Design review of the part built by this model. Coordinates are the model's own, in mm. A direction names the side the tool comes from. Give positions to 0.01 mm unless a question says otherwise; leave off trailing zeros. Write each question's results on one line, items separated by ' | '. Start each with the question number.
from build123d import *

# Parameters (mm, degrees)
BOSS_EXTRUDE1_DEPTH = 3.175
BOSS_EXTRUDE2_DEPTH = 3.175
BOSS_EXTRUDE3_DEPTH = 3.175


with BuildPart() as part:
    # Sketch1 → Boss-Extrude1 (new body)
    with BuildSketch(Plane.XY):
        with BuildLine():
            Line((0, 0), (0, 35.921024484))
            ThreePointArc((0, 35.921024484), (-25.4, 25.4), (-35.921024484, 0))
            Line((-35.921024484, 0), (0, 0))
        make_face()
    extrude(amount=BOSS_EXTRUDE1_DEPTH)

    # Sketch2 → Boss-Extrude2 (add)
    with BuildSketch(Plane(origin=(0, 0, 0), x_dir=(0, 0, -1), z_dir=(1, 0, 0))):
        with BuildLine():
            Line((0, 0), (25.4, 0))
            Line((25.4, 0), (25.4, 17.145))
            ThreePointArc((25.4, 17.145), (15.793187578, 30.717442473), (0, 35.921024484))
            Line((0, 35.921024484), (-3.175, 35.921024484))
            Line((-3.175, 35.921024484), (-3.175, 0))
            Line((-3.175, 0), (0, 0))
        make_face()
    extrude(amount=BOSS_EXTRUDE2_DEPTH)

    # Sketch3 → Boss-Extrude3 (add)
    with BuildSketch(Plane.XZ):
        with BuildLine():
            Line((0, -25.4), (-17.145, -25.4))
            ThreePointArc((-17.145, -25.4), (-30.717442473, -15.793187578), (-35.921024484, 0))
            Line((-35.921024484, 0), (-35.921024484, 3.175))
            Line((-35.921024484, 3.175), (3.175, 3.175))
            Line((3.175, 3.175), (3.175, -25.4))
            Line((3.175, -25.4), (0, -25.4))
        make_face()
    extrude(amount=BOSS_EXTRUDE3_DEPTH)

    # Chamfer1
    # the kernel refuses this chamfer: 2.032 mm, written as the material it takes off along each edge
    with BuildSketch(Plane(origin=(1.820333333, 34.566357818, 1.820333333), x_dir=(0, -0.7071067811865468, 0.7071067811865481), z_dir=(0.5773502691896253, 0.5773502691896264, 0.5773502691896256))) as chamfer1_piece_1:
        Polygon((-1.436840979, -0.829560526), (1.436840979, -0.829560526), (0, 1.659121052), align=None)
    extrude(amount=2.580986643, mode=Mode.SUBTRACT)
    with BuildSketch(Plane(origin=(1.820333333, -1.820333333, -24.045333333), x_dir=(-0.7071067811865476, 0, -0.7071067811865476), z_dir=(0.5773502691896256, -0.577350269189626, -0.5773502691896256)), Plane(origin=(1.820333333, -1.820333333, 1.820333333), x_dir=(0.7071067811865476, 0, -0.7071067811865474), z_dir=(0.5773502691896254, -0.577350269189626, 0.577350269189626)), Plane(origin=(-34.566357818, -1.820333333, 1.820333333), x_dir=(0.7071067811865468, 0, 0.7071067811865481), z_dir=(-0.5773502691896263, -0.5773502691896255, 0.5773502691896255))) as chamfer1_piece_2:
        Polygon((-1.436840979, 0.829560526), (1.436840979, 0.829560526), (0, -1.659121052), align=None)
    extrude(amount=2.580986643, mode=Mode.SUBTRACT)
    with BuildSketch(Plane(origin=(0, 0, 3.175), x_dir=(0, 1, 0), z_dir=(1, 0, 0))) as chamfer1_piece_3:
        with BuildLine():
            Line((35.978498123, -2.089473639), (33.831550845, 0.057473639))
            Line((33.831550845, 0.057473639), (33.831550845, 0.098113639))
            ThreePointArc((33.831550845, 0.098113639), (34.876287665, 0.04064), (35.921024484, 0.04064))
            Line((35.921024484, 0.04064), (35.961664484, 0))
            ThreePointArc((35.961664484, 0), (35.961664484, -1.04473682), (36.019138123, -2.089473639))
            Line((36.019138123, -2.089473639), (35.978498123, -2.089473639))
        make_face()
    revolve(axis=Axis((0, 0, 3.175), (0, 0, 1)), revolution_arc=90, mode=Mode.SUBTRACT)
    with BuildSketch(Plane(origin=(0, 35.921024484, 3.175), x_dir=(0, -0.9996219169112968, 0.027495876610586455), z_dir=(1, 0, 0)), Plane(origin=(-35.921024484, -3.175, 0), x_dir=(0.9996219169112968, -0.027495876610586455, 0), z_dir=(0, 0, 1))) as chamfer1_piece_4:
        with BuildLine():
            Line((2.090263933, 0), (-0.114903819, 2.087103356))
            Line((-0.114903819, 2.087103356), (-0.155528453, 2.085985924))
            ThreePointArc((-0.155528453, 2.085985924), (-0.069350589, 1.04322439), (-0.040624635, -0.001117432))
            Line((-0.040624635, -0.001117432), (0.001117432, -0.040624635))
            ThreePointArc((0.001117432, -0.040624635), (1.045459255, -0.01189868), (2.091381365, -0.040624635))
            Line((2.091381365, -0.040624635), (2.090263933, 0))
        make_face()
    extrude(amount=8.400659832, mode=Mode.SUBTRACT)
    with BuildSketch(Plane(origin=(3.175, 22.370659832, -25.4), x_dir=(0.027495876610586455, 0, 0.9996219169112968), z_dir=(0, -1, 0))) as chamfer1_piece_5:
        with BuildLine():
            Line((2.090263933, 0), (-0.114903819, 2.087103356))
            Line((-0.114903819, 2.087103356), (-0.155528453, 2.085985924))
            ThreePointArc((-0.155528453, 2.085985924), (-0.069350589, 1.04322439), (-0.040624635, -0.001117432))
            Line((-0.040624635, -0.001117432), (0.001117432, -0.040624635))
            ThreePointArc((0.001117432, -0.040624635), (1.045459255, -0.01189868), (2.091381365, -0.040624635))
            Line((2.091381365, -0.040624635), (2.090263933, 0))
        make_face()
    extrude(amount=30.771319663, mode=Mode.SUBTRACT)
    with BuildSketch(Plane(origin=(3.175, 9.352591527, 0), x_dir=(0, 0.1007624019843993, -0.9949105177584235), z_dir=(0, -0.9949105177584235, -0.1007624019843993))) as chamfer1_piece_6:
        with BuildLine():
            Line((24.478959318, 0.057473639), (26.625906597, -2.089473639))
            Line((26.625906597, -2.089473639), (26.666546597, -2.089473639))
            ThreePointArc((26.666546597, -2.089473639), (26.609072957, -1.04473682), (26.609072957, 0))
            Line((26.609072957, 0), (26.568432957, 0.04064))
            ThreePointArc((26.568432957, 0.04064), (25.523696138, 0.04064), (24.478959318, 0.098113639))
            Line((24.478959318, 0.098113639), (24.478959318, 0.057473639))
        make_face()
    revolve(axis=Axis((3.175, 9.352591527, 0), (1, 0, 0)), revolution_arc=84.216925348, mode=Mode.SUBTRACT)
    with BuildSketch(Plane(origin=(3.175, 35.921024484, 0), x_dir=(0.027495876610586455, -0.9996219169112968, 0), z_dir=(0, 0, 1)), Plane(origin=(-35.921024484, 0, 3.175), x_dir=(0.9996219169112968, 0, 0.027495876610586455), z_dir=(0, -1, 0))) as chamfer1_piece_7:
        with BuildLine():
            Line((2.090263933, 0), (-0.114903819, -2.087103356))
            Line((-0.114903819, -2.087103356), (-0.155528453, -2.085985924))
            ThreePointArc((-0.155528453, -2.085985924), (-0.069350589, -1.04322439), (-0.040624635, 0.001117432))
            Line((-0.040624635, 0.001117432), (0.001117432, 0.040624635))
            ThreePointArc((0.001117432, 0.040624635), (1.045459255, 0.01189868), (2.091381365, 0.040624635))
            Line((2.091381365, 0.040624635), (2.090263933, 0))
        make_face()
    extrude(amount=8.400659832, mode=Mode.SUBTRACT)
    with BuildSketch(Plane(origin=(3.175, -8.400659832, 3.175), x_dir=(-0.9996219169112968, 0, 0.027495876610586435), z_dir=(0, 1, 0)), Plane(origin=(-41.146684316, -3.175, 3.175), x_dir=(0, 0.9996219169112968, 0.027495876610586435), z_dir=(1, 0, 0))) as chamfer1_piece_8:
        with BuildLine():
            Line((2.090263933, 0), (-0.114903819, -2.087103356))
            Line((-0.114903819, -2.087103356), (-0.155528453, -2.085985924))
            ThreePointArc((-0.155528453, -2.085985924), (-0.069350589, -1.04322439), (-0.040624635, 0.001117432))
            Line((-0.040624635, 0.001117432), (0.001117432, 0.040624635))
            ThreePointArc((0.001117432, 0.040624635), (1.045459255, 0.01189868), (2.091381365, 0.040624635))
            Line((2.091381365, 0.040624635), (2.090263933, 0))
        make_face()
    extrude(amount=49.547344147, mode=Mode.SUBTRACT)
    with BuildSketch(Plane(origin=(8.400659832, -3.175, -25.4), x_dir=(0, 0.9996219169112968, -0.027495876610585585), z_dir=(-1, 0, 0))) as chamfer1_piece_9:
        with BuildLine():
            Line((2.090263933, 0), (-0.114903819, -2.087103356))
            Line((-0.114903819, -2.087103356), (-0.155528453, -2.085985924))
            ThreePointArc((-0.155528453, -2.085985924), (-0.069350589, -1.04322439), (-0.040624635, 0.001117432))
            Line((-0.040624635, 0.001117432), (0.001117432, 0.040624635))
            ThreePointArc((0.001117432, 0.040624635), (1.045459255, 0.01189868), (2.091381365, 0.040624635))
            Line((2.091381365, 0.040624635), (2.090263933, 0))
        make_face()
    extrude(amount=30.771319663, mode=Mode.SUBTRACT)
    with BuildSketch(Plane(origin=(3.175, -3.175, 8.400659832), x_dir=(0.027495876610586435, 0.9996219169112968, 0), z_dir=(0, 0, -1))) as chamfer1_piece_10:
        with BuildLine():
            Line((2.090263933, 0), (-0.114903819, -2.087103356))
            Line((-0.114903819, -2.087103356), (-0.155528453, -2.085985924))
            ThreePointArc((-0.155528453, -2.085985924), (-0.069350589, -1.04322439), (-0.040624635, 0.001117432))
            Line((-0.040624635, 0.001117432), (0.001117432, 0.040624635))
            ThreePointArc((0.001117432, 0.040624635), (1.045459255, 0.01189868), (2.091381365, 0.040624635))
            Line((2.091381365, 0.040624635), (2.090263933, 0))
        make_face()
    extrude(amount=39.026319663, mode=Mode.SUBTRACT)
    with BuildSketch(Plane(origin=(-9.352591527, -3.175, 0), x_dir=(-0.1007624019843981, 0, -0.9949105177584237), z_dir=(0.9949105177584237, 0, -0.1007624019843981))) as chamfer1_piece_11:
        with BuildLine():
            Line((26.625906597, 2.089473639), (24.478959318, -0.057473639))
            Line((24.478959318, -0.057473639), (24.478959318, -0.098113639))
            ThreePointArc((24.478959318, -0.098113639), (25.523696138, -0.04064), (26.568432957, -0.04064))
            Line((26.568432957, -0.04064), (26.609072957, 0))
            ThreePointArc((26.609072957, 0), (26.609072957, 1.04473682), (26.666546597, 2.089473639))
            Line((26.666546597, 2.089473639), (26.625906597, 2.089473639))
        make_face()
    revolve(axis=Axis((-9.352591527, -3.175, 0), (0, 1, 0)), revolution_arc=84.216925348, mode=Mode.SUBTRACT)


solid = part.part
Q1. For pin 1 Ø3 at (x, z) = (-3, -21.5) entering from +Y; pin 2 Ø1 at (x, y) = (-22, 26) entering from -Z, all flat-tipped, find the tip position at first contact; note any pin that passes through.
Q2. For faces 1 (the flat face through (2.173, 34.891, 0.563)), 2 (the flat face through (0, 14, -13)), list the 3-axis set-ups (+Z, -Z, +X, -X, +Y, -Y) from which the entire face can be reached by the end or side of a thin tool; tool diameter is ignored.
Q3. Wall thickness on line 1 along Y through (x, z) = (-2, -12) (3 decimals); line 2 along X through (y, z) = (17, -19) (3 decimals): over which ranges is each line inside the solid? List them lowest first. Write a range as from..to.
Answer sheet:
1) pin 1: y = 0 | pin 2: z = 0
2) face 1: +Z, -Z, +X, +Y | face 2: -Z, -X, +Y
3) line 1: -3.175..0 | line 2: 0..3.175
